Part model, mm, in its own coordinate system. Face numbers are marked on the shaded views. A direction names the side the tool comes from. Round coordinates to 2 decimals unless told otherwise and drop trailing zeros. Write each loop counter-clockwise with the first axis right and the second up, starting at its lowest first coordinate (ties: lowest second). Pieces come first, ordered by that corner, then holes. Notation, with made-up numbers: M 59.5,-15 L 66.5,-15 A12 cw 66.5,-9 Z; hole C 45.25,17 d7. An arc over 180 degrees is marked long. One line per question, with ' | ' between items. Start each with the question number.
1) Saw through at C-C (z = 10). List the corners of the cut face in (x, y), plus the area to 3 significant figures.
2) Wall check: probe 1 along X at (y, z) = (20.5, 17.25); probe 2 along Y at (x, z) = (-46.75, 8.5); probe 3 along Y at (x, z) = (-54, 11). Give the ranges that are in metal, low to high. Write a range as [from, to].
3) Saw through at B-B (y = 19.75). List the corners of the cut face in (x, z), plus the area to 3 significant figures.
4) Drop flat-ended pins along their axis: pin 1 Ø0.9 at (x, z) = (-27, 11) entering from +Y; pin 2 Ø3.5 at (y, z) = (22.31, 10) entering from -X; pin 3 Ø5 at (y, z) = (15.5, 18) entering from +X. Give the stop position or say it passes through.
5) Saw through at D-D (y = 22.75). List the corners of the cut face in (x, z), plus the area to 3 significant figures.
6) Tool access for the marked faces 5, 6, 7 and 8: list every direction of +Z, -Z, +X, -X, +Y, -Y with a clear straight run to the whole face (end or side of a thin tool).
7) Mould opens along Y. For the marked faces 1, 2, 3 and 4 say: pulls with the +Y half, pulls with the -Y half, needs draft (parallel to the pull), parting line crosses it, or undercut.
8) Saw through at A-A (x = -41.5). List the corners of the cut face in (y, z).
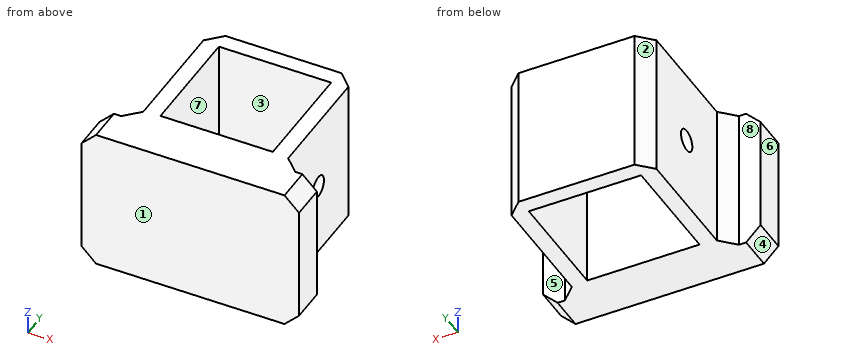
```python
from build123d import *

# Parameters (mm, degrees)
F0_W     = 20
F0_H     = 20
F0_W_2   = 15.5
F0_H_2   = 15.5
F1_DEPTH = 20
F2_SIZE  = 2
F3_R     = 1.5
F4_DEPTH = 25


with BuildPart() as f1:
    # F0 (on Top) → F1 (new body)
    with BuildSketch(Plane.XY):
        with Locations((-40.922806, 22.305217)):
            Rectangle(F0_W, F0_H)
        with Locations((-40.922806, 22.305217)):
            Rectangle(F0_W_2, F0_H_2, mode=Mode.SUBTRACT)
        Polygon((-30.922806, 12.305217), (-50.922806, 12.305217), (-55.922806, 12.305217), (-55.922806, 7.555217), (-25.922806, 7.555217), (-25.922806, 12.305217), align=None)
    extrude(amount=F1_DEPTH)

    # F2
    f2_edges = [f1.edges().sort_by_distance(p)[0] for p in [
        (-50.922806, 32.305217, 10),
        (-30.922806, 32.305217, 10),
        (-25.922806, 9.930217, 20),
        (-55.922806, 9.930217, 20),
        (-55.922806, 9.930217, 0),
        (-25.922806, 9.930217, 0),
        (-30.922806, 12.305217, 10),
        (-50.922806, 12.305217, 10),
    ]]
    chamfer(f2_edges, length=F2_SIZE)

    # F3 (on face) → F4 (cut)
    with BuildSketch(Plane(origin=(-50.922806, 0, 0), x_dir=(0, -1, 0), z_dir=(-1, 0, 0))):
        with Locations((-22.305217, 10)):
            Circle(F3_R)
    extrude(amount=-F4_DEPTH, mode=Mode.SUBTRACT)


solid = f1.part
```
Answer key:
1) outline: M -55.92,7.56 L -25.92,7.56 L -25.92,12.31 L -28.92,12.31 L -30.92,14.31 L -30.92,20.81 L -33.17,20.81 L -33.17,14.56 L -48.67,14.56 L -48.67,20.81 L -50.92,20.81 L -50.92,14.31 L -52.92,12.31 L -55.92,12.31 Z; M -50.92,23.81 L -48.67,23.81 L -48.67,30.06 L -33.17,30.06 L -33.17,23.81 L -30.92,23.81 L -30.92,30.31 L -32.92,32.31 L -48.92,32.31 L -50.92,30.31 Z | area: 289 mm2
2) probe 1: x = [-50.92, -48.67], [-33.17, -30.92] | probe 2: y = [7.56, 14.56], [30.06, 32.31] | probe 3: y = [7.56, 12.31]
3) outline: M -50.92,0 L -48.67,0 L -48.67,20 L -50.92,20 Z; M -33.17,0 L -30.92,0 L -30.92,20 L -33.17,20 Z | area: 90.0 mm2
4) pin 1: stops at y = 12.31 | pin 2: stops at x = -50.92 | pin 3: stops at x = -29.62
5) outline: M -50.92,0 L -48.67,0 L -48.67,8.57 L -50.92,8.57 Z; M -50.92,11.43 L -48.67,11.43 L -48.67,20 L -50.92,20 Z; M -33.17,0 L -30.92,0 L -30.92,8.57 L -33.17,8.57 Z; M -33.17,11.43 L -30.92,11.43 L -30.92,20 L -33.17,20 Z | area: 77.1 mm2
6) face 5: +Z, -Z, +X, +Y | face 6: +Z, -Z, -X, +Y, -Y | face 7: +Z, -Z | face 8: +Z, -Z, -X, +Y
7) face 1: pulls with the -Y half | face 2: pulls with the +Y half | face 3: undercut | face 4: needs draft
8) outline: M 7.56,0 L 14.56,0 L 14.56,20 L 7.56,20 Z; M 30.06,0 L 32.31,0 L 32.31,20 L 30.06,20 Z
